from build123d import *

# Parameters (mm, degrees)
CUT_EXTRUDE1_DEPTH = 4


with BuildPart() as part:
    # Sketch1 → Revolve1 (revolve)
    with BuildSketch(Plane(origin=(0, 0, 0), x_dir=(1, 0, 0), z_dir=(0, 1, 0))):
        with BuildLine():
            Line((0, 0), (0, -15))
            Line((0, -15), (5, -20))
            Line((5, -20), (30, -20))
            Line((30, -20), (30, -26))
            Line((30, -26), (35, -26))
            Line((35, -26), (35, -20))
            Line((35, -20), (105, -20))
            Line((105, -20), (105, -17))
            Line((105, -17), (216, -17))
            Line((216, -17), (216, -15))
            Line((216, -15), (216, -14.1))
            ThreePointArc((216, -14.1), (216.46862915, -12.96862915), (217.6, -12.5))
            Line((217.6, -12.5), (220.585786438, -12.5))
            ThreePointArc((220.585786438, -12.5), (220.96846987, -12.576120467), (221.292893219, -12.792893219))
            Line((221.292893219, -12.792893219), (223.5, -15))
            Line((223.5, -15), (252.5, -15))
            Line((252.5, -15), (255, -12.5))
            Line((255, -12.5), (255, 0))
            Line((255, 0), (0, 0))
        make_face()
    revolve(axis=Axis((-87.77690163, 0, 0), (1, 0, 0)))

    # Sketch5 → Cut-Revolve1 (revolve, cut)
    with BuildSketch(Plane.ZY.offset(-15)):
        Polygon((20, 0), (20, 3), (17, 0), align=None)
    revolve(axis=Axis((15, 0, 17), (0, 0, 1)), mode=Mode.SUBTRACT)

    # Sketch6 → Cut-Extrude1 (cut)
    with BuildSketch(Plane(origin=(0, 0, -20), x_dir=(-1, 0, 0), z_dir=(0, 0, -1))):
        with BuildLine():
            Line((-73, 6), (-53, 6))
            ThreePointArc((-53, 6), (-47, 0), (-53, -6))
            Line((-53, -6), (-73, -6))
            ThreePointArc((-73, -6), (-79, 0), (-73, 6))
        make_face()
    extrude(amount=-CUT_EXTRUDE1_DEPTH, mode=Mode.SUBTRACT)


solid = part.part
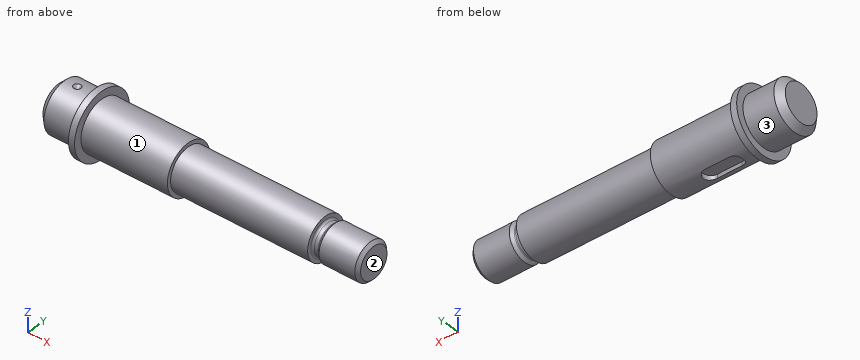
CAD build for the part. Positions are in the model's coordinates, mm. Face numbers are marked on the shaded views. A direction names the side the tool comes from. Round coordinates to 2 decimals unless told otherwise and drop trailing zeros. Loops run counter-clockwise (first coordinate to the right, second up) from the corner with the lowest first, then second, coordinate; pieces in that order, holes last.
(1) Cut at C-C (x = 134). Give the cut face in (y, z), plus the area to 3 significant figures.
(2) Drop flat-ended pins along their axis: pin 1 (6 mm diameter, centred on x = 65.5, y = 2.5, fed in from -Z); pin 2 (3.5 mm diameter, centred on x = 65, z = -17.5, fed in from +Y); pin 3 (8 mm diameter, centred on x = 90.5, z = 2.5, fed in from -Y); pin 4 (10 mm diameter, centred on y = 7, z = -11, fed in from +X). Give the stop position or say it passes through.
(3) Cut at B-B (x = 37.5). Give the cut face in (y, z).
(4) Wall check: line 1 along Z through (x, y) = (30.5, -1); line 2 along Y through (x, z) = (27, -0.5); line 3 along X through (y, z) = (20.5, -1). Give the ranges that are in metal, low to high.
(5) Which spindle directions (+Z, -Z, +X, -X, +Y, -Y) get a long thin tool onto all of the face, cutting with end or side? Do the marked faces 1, 2 and 3. Say none if no direction does.
(6) Cut at D-D (x = 64.5). Give the cut face in (y, z), plus the area to 3 significant figures.
Findings below:
1. outline: circle Ø34 at (0, 0)
1. area: 908 mm2
2. pin 1: stops at z = -16
2. pin 2: stops at y = 12.33
2. pin 3: stops at y = -20
2. pin 4: stops at x = 255
3. outline: circle Ø40 at (0, 0)
4. line 1: z = -25.98 to 25.98
4. line 2: y = -19.99 to 19.99
4. line 3: x = 30 to 35
5. face 1: +X
5. face 2: +Z, -Z, +X, +Y, -Y
5. face 3: -X
6. outline: (-6, -19.08) - (-6, -16) - (6, -16) - (6, -19.08) arc R20 ccw (long way) to start
6. area: 1,210 mm2
